from build123d import *

# Parameters (mm, degrees)
F0_R          = 3.3
F0_R_2        = 2.5
F1_DEPTH      = 5
F2_DEPTH      = 5
F2_DEPTH_BACK = 21.8
F5_R          = 3.25
F5_R_2        = 2.5
F6_DEPTH      = 6
F7_W          = 59.1
F7_H          = 2
F7_W_2        = 6
F8_DEPTH      = 1
F7_W_3        = 13.4
F9_DEPTH      = 6
F10_DEPTH     = 30
F11_R         = 2


with BuildPart() as f1:
    # F0 (on Front) → F1 (new body)
    with BuildSketch(Plane.XZ):
        with BuildLine():
            Line((13.9969279973, 24), (0, 24))
            Line((0, 24), (0, 0))
            Line((0, 0), (14.3809281676, 0))
            ThreePointArc((14.3809281676, 0), (25.9984639003, 12.1889526569), (13.9969279973, 24))
        make_face()
        with Locations((15, 11.9969279973)):
            Circle(F0_R, mode=Mode.SUBTRACT)
        with Locations((15, 11.9969279973)):
            Circle(F0_R)
        with Locations((15, 11.9969279973)):
            Circle(F0_R_2, mode=Mode.SUBTRACT)
    extrude(amount=F1_DEPTH)

    # F0 (on Front) → F2 (join, two sides)
    with BuildSketch(Plane.XZ) as f2_sk:
        Polygon((0, 0), (0, 24), (0, 24.0955166519), (-5, 24.0955166519), (-5, 0), align=None)
    extrude(amount=F2_DEPTH)
    extrude(f2_sk.sketch, amount=-F2_DEPTH_BACK)

    # F4: F1 across plane


with BuildPart() as f1_1:
    add(f1.part)
    add(f1.part.mirror(Plane.XZ.offset(-8.4)))

    # F5 (on face) → F6 (cut)
    with BuildSketch(Plane(origin=(0, 21.8, 0), x_dir=(-1, 0, 0), z_dir=(0, 1, 0))):
        with Locations((-15, 11.9969279973)):
            Circle(F5_R)
        with Locations((-15, 11.9969279973)):
            Circle(F5_R_2, mode=Mode.SUBTRACT)
    extrude(amount=-F6_DEPTH, mode=Mode.SUBTRACT)

    # F7 (on face) → F8 (join)
    with BuildSketch(Plane(origin=(-5, 0, 0), x_dir=(0, -1, 0), z_dir=(-1, 0, 0))):
        with Locations((-51.35, 1)):
            Rectangle(F7_W, F7_H)
        with Locations((34.55, 1)):
            Rectangle(F7_W, F7_H)
        Polygon((-86.9, 0), (-80.9, 0), (-80.9, 2), (-86.9, 2), (-86.9, 1), align=None)
        Polygon((-80.9, 2), (-21.8, 2), (-21.8, 7.25), (-86.9, 7.25), (-86.9, 2), align=None)
        Polygon((5, 12.5), (5, 2), (64.1, 2), (70.1, 2), (70.1, 7.25), (70.1, 12.5), (64.1, 12.5), align=None)
        Polygon((64.1, 2), (64.1, 0), (70.1, 0), (72.1, 0), (72.1, 7.25), (72.1, 14.5), (70.1, 14.5), (70.1, 12.5), (70.1, 7.25), (70.1, 2), align=None)
        Polygon((-88.9, 0), (-86.9, 0), (-86.9, 1), (-86.9, 2), (-86.9, 7.25), (-88.9, 7.25), align=None)
        Polygon((-86.9, 7.25), (-21.8, 7.25), (-21.8, 12.5), (-80.9, 12.5), (-86.9, 12.5), align=None)
        with Locations((34.55, 13.5)):
            Rectangle(F7_W, F7_H)
        Polygon((-88.9, 7.25), (-86.9, 7.25), (-86.9, 12.5), (-86.9, 14.5), (-88.9, 14.5), align=None)
        with Locations((-51.35, 13.5)):
            Rectangle(F7_W, F7_H)
        with Locations((67.1, 13.5)):
            Rectangle(F7_W_2, F7_H)
        with Locations((-83.9, 13.5)):
            Rectangle(F7_W_2, F7_H)
    extrude(amount=-F8_DEPTH)

    # F7 (on face) → F9 (join)
    with BuildSketch(Plane(origin=(-5, 0, 0), x_dir=(0, -1, 0), z_dir=(-1, 0, 0))):
        with Locations((34.55, 13.5)):
            Rectangle(F7_W, F7_H)
        with Locations((67.1, 13.5)):
            Rectangle(F7_W_2, F7_H)
        Polygon((64.1, 2), (64.1, 0), (70.1, 0), (72.1, 0), (72.1, 7.25), (72.1, 14.5), (70.1, 14.5), (70.1, 12.5), (70.1, 7.25), (70.1, 2), align=None)
        with Locations((34.55, 1)):
            Rectangle(F7_W, F7_H)
        with Locations((-15.1, 1)):
            Rectangle(F7_W_3, F7_H)
        with Locations((-1.7, 1)):
            Rectangle(F7_W_3, F7_H)
        Polygon((-8.4, 12.5), (5, 12.5), (5, 14.5), (-8.4, 14.5), (-21.8, 14.5), (-21.8, 12.5), align=None)
        with Locations((-51.35, 13.5)):
            Rectangle(F7_W, F7_H)
        with Locations((-51.35, 1)):
            Rectangle(F7_W, F7_H)
        with Locations((-83.9, 13.5)):
            Rectangle(F7_W_2, F7_H)
        Polygon((-88.9, 7.25), (-86.9, 7.25), (-86.9, 12.5), (-86.9, 14.5), (-88.9, 14.5), align=None)
        Polygon((-88.9, 0), (-86.9, 0), (-86.9, 1), (-86.9, 2), (-86.9, 7.25), (-88.9, 7.25), align=None)
        Polygon((-86.9, 0), (-80.9, 0), (-80.9, 2), (-86.9, 2), (-86.9, 1), align=None)
    extrude(amount=F9_DEPTH)

    # F7 (on face) → F10 (join)
    with BuildSketch(Plane(origin=(-5, 0, 0), x_dir=(0, -1, 0), z_dir=(-1, 0, 0))):
        with Locations((-83.9, 13.5)):
            Rectangle(F7_W_2, F7_H)
        Polygon((-88.9, 7.25), (-86.9, 7.25), (-86.9, 12.5), (-86.9, 14.5), (-88.9, 14.5), align=None)
        Polygon((-88.9, 0), (-86.9, 0), (-86.9, 1), (-86.9, 2), (-86.9, 7.25), (-88.9, 7.25), align=None)
        Polygon((-86.9, 0), (-80.9, 0), (-80.9, 2), (-86.9, 2), (-86.9, 1), align=None)
        Polygon((64.1, 2), (64.1, 0), (70.1, 0), (72.1, 0), (72.1, 7.25), (72.1, 14.5), (70.1, 14.5), (70.1, 12.5), (70.1, 7.25), (70.1, 2), align=None)
        with Locations((67.1, 13.5)):
            Rectangle(F7_W_2, F7_H)
    extrude(amount=F10_DEPTH)

    # F11
    f11_edges = [f1_1.edges().sort_by_distance(p)[0] for p in [
        (-20, -70.1, 12.5),
        (-5, 8.4, 12.5),
        (-20, 86.9, 12.5),
    ]]
    fillet(f11_edges, radius=F11_R)


solid = f1_1.part
Could you check a few things on this model? Use its own coordinates, in mm. A direction names the side the tool comes from. Give positions to 0.01 mm unless a question says otherwise; leave off trailing zeros. Order: outer loops, then holes, each group sorted by start corner. A loop starts at its lowest first (then second) coordinate and runs counter-clockwise, first axis right, second up. Notation, with made-up numbers: (11.5, -32) - (61.5, -32) arc R19 ccw to (61.5, -9) - close; hole circle Ø6 at (52, -28). An arc over 180 degrees is marked (long way). One line per question, with ' | ' between items. Start each with the question number.
Item 1: For faces 4 (the flat face through (-20, 86.9, 6)), 5 (the flat face through (10, 0, 12)), 6 (the flat face through (-4, -38, 7)), which set-ups out of +Z, -Z, +X, -X, +Y, -Y let a thin tool reach every point of the face, with its end or its side?
Item 2: I want a section at A-A on x = -12.5. Write out the boundary of the cut face in (y, z), then the cut area to 3 significant figures.
Item 3: I'm going to push flat-ended pins straight in: pin 1 Ø1.5 at (x, z) = (7.5, 5) entering from -Y; pin 2 Ø12 at (y, z) = (1, 21.5) entering from +X; pin 3 Ø12 at (y, z) = (8, 17) entering from +X; pin 4 Ø6 at (x, y) = (16.5, 21) entering from -Z. Where does each tip first touch, or does it pass through?
Item 4: I want a section at D-D on y = 43.5. Write out the boundary of the cut face in (x, z), then the cut area to 3 significant figures.
Item 5: I need wall thicknesses on probe 1 along Y at (x, z) = (23, 16.75); probe 2 along Y at (x, z) = (-19.5, 8); probe 3 along Z at (x, y) = (-9.5, -19.5). Which ranges of each line are inside material? Lowest first, please. Write a range as [from, to].
Item 6: I want a section at B-B on y = 8.5. Write out the boundary of the cut face in (x, z), then the cut area to 3 significant figures.
Item 7: I want a section at C-C on z = 5. Write out the boundary of the cut face in (x, y), then the cut area to 3 significant figures.
Item 8: Thinking about a two-plate mould opening in X: for faces 1 (the cylindrical face through (26, 19, 12)), 2 (the cylindrical face through (18.247, 19.335, 12.14)), 3 (the flat face through (-19, -72.1, 7)), which applies, pulls with the +X half, pulls with the -X half, needs draft (parallel to the pull), parting line crosses it, or undercut?
Verdict:
1) face 4: -X | face 5: +Z, -Z, +X | face 6: +Z, -Z, +X, -Y
2) outline: (-72.1, 0) - (-64.1, 0) - (-64.1, 2) - (-70.1, 2) - (-70.1, 10.5) arc R2 cw to (-68.1, 12.5) - (-64.1, 12.5) - (-64.1, 14.5) - (-72.1, 14.5) - close; (80.9, 0) - (88.9, 0) - (88.9, 14.5) - (80.9, 14.5) - (80.9, 12.5) - (84.9, 12.5) arc R2 cw to (86.9, 10.5) - (86.9, 2) - (80.9, 2) - close | area: 108 mm^2
3) pin 1: y = -5 | pin 2: x = 25.45 | pin 3: x = 0 | pin 4: z = 0
4) outline: (-11, 0) - (-4, 0) - (-4, 14.5) - (-11, 14.5) - (-11, 12.5) - (-7, 12.5) arc R2 cw to (-5, 10.5) - (-5, 2) - (-11, 2) - close | area: 39.4 mm^2
5) probe 1: [-5, 0], [16.8, 21.8] | probe 2: [-72.1, -70.1], [86.9, 88.9] | probe 3: [0, 2], [12.5, 14.5]
6) outline: (-11, 0) - (0, 0) - (0, 24.1) - (-5, 24.1) - (-5, 14.5) - (-11, 14.5) - (-11, 12.5) - (-7, 12.5) arc R2 cw to (-5, 10.5) - (-5, 2) - (-11, 2) - close | area: 145 mm^2
7) outline: (-35, -72.1) - (-4, -72.1) - (-4, -5) - (23.75, -5) - (23.75, 0) - (0, 0) - (0, 16.8) - (23.75, 16.8) - (23.75, 21.8) - (-4, 21.8) - (-4, 88.9) - (-35, 88.9) - (-35, 86.9) - (-5, 86.9) - (-5, -70.1) - (-35, -70.1) - close | area: 626 mm^2
8) face 1: pulls with the +X half | face 2: undercut | face 3: needs draft
